Can you work these out from the model? Positions are in its coordinate system, mm. A direction names the side the tool comes from. Give positions to 0.01 mm unless a question says otherwise; leave off trailing zeros. Write each loop counter-clockwise with the first axis right and the second up, starting at its lowest first coordinate (ties: lowest second). Pieces come first, ordered by that corner, then holes. Notation, with made-up numbers: (62, 7.25) -> (119, 7.25) arc R33 ccw to (119, 45.25) -> close; hole circle Ø3 at (15.25, 20.25). An arc over 180 degrees is marked (long way). Answer as CSV lines item,"result". Start each with the question number.
1. If we mould it in two halves opening along X, with no side actions, what happens to faces 3 (the face through (66, 3, -50.8)), 4 (the face through (75.5, 3.1, 0.7)), 5 (the face through (3.175, 3, -13))? For each: pulls with the +X half, pulls with the -X half, needs draft (parallel to the pull), parting line crosses it, or undercut.
2. If we section it at A-A on z = 4.5: Write out the boundary of the cut face in (x, y) (3 decimals), plus the area to 3 significant figures.
3. I need wall thicknesses on line 1 (X direction, y = 5.75, z = 7.5) (3 decimals); line 2 (X direction, y = 5.5, z = -15) (3 decimals); line 3 (X direction, y = 3, z = 38). Which ranges of each line are inside material? Lowest first, please. Write a range as [from, to].
4. I'm going to push flat-ended pins straight in: P1, Ø3, axis at y = 4, z = -20, coming from the +X side; P2, Ø1.5, axis at y = 1, z = 34.5, coming from the +X side; P3, Ø1.9, axis at y = 3.5, z = -27, coming from the -X side. Where does each tip first touch, or does it pass through?
5. If we section it at D-D on x = -97: Write out the boundary of the cut face in (y, z), plus the area to 4 significant figures.
6. On a 3-axis mill with a long thin cutter (end or side, diameter ignored), from which of +Z, -Z, +X, -X, +Y, -Y can I reach the whole of each face in a straight line? I mean faces 1 (the face through (-3.175, 3, -12)), 2 (the face through (-26, 6.35, -12)). Say none if no direction works.
7. If we section it at B-B on y = 5: Write out the boundary of the cut face in (x, z) (3 decimals).
8. If we section it at C-C on z = -38.5: Write out the boundary of the cut face in (x, y) (3 decimals).
```python
from build123d import *

# Parameters (mm, degrees)
BOSS_EXTRUDE1_DEPTH = 6.35


with BuildPart() as part:
    # Sketch1 → Boss-Extrude1 (new body)
    with BuildSketch(Plane(origin=(0, 0, 0), x_dir=(1, 0, 0), z_dir=(0, 1, 0))):
        Polygon((-127, 50.8), (-25.4, 50.8), (-25.4, -50.8), align=None)
        with BuildLine():
            Line((-25.4, 50.8), (-25.4, -50.8))
            Line((-25.4, -50.8), (25.4, -50.8))
            Line((25.4, -50.8), (25.4, 50.8))
            Line((25.4, 50.8), (3.175, 50.8))
            Line((3.175, 50.8), (3.175, -25.4))
            ThreePointArc((3.175, -25.4), (0, -28.575), (-3.175, -25.4))
            Line((-3.175, -25.4), (-3.175, 50.8))
            Line((-3.175, 50.8), (-25.4, 50.8))
        make_face()
        Polygon((25.4, -50.8), (127, 50.8), (25.4, 50.8), align=None)
    extrude(amount=BOSS_EXTRUDE1_DEPTH)


solid = part.part
```
Computed values:
1,face 3,"needs draft"
1,face 4,"pulls with the +X half"
1,face 5,"undercut"
2,outline,"(-71.7, 0) -> (-3.175, 0) -> (-3.175, 6.35) -> (-71.7, 6.35) -> close; (3.175, 0) -> (71.7, 0) -> (71.7, 6.35) -> (3.175, 6.35) -> close"
2,area,"870 mm2"
3,line 1,"x = [-68.7, -3.175], [3.175, 68.7]"
3,line 2,"x = [-91.2, -3.175], [3.175, 91.2]"
3,line 3,"x = [-38.2, 38.2]"
4,P1,"stops at x = 97.7"
4,P2,"stops at x = 42.45"
4,P3,"stops at x = -104.15"
5,outline,"(0, -50.8) -> (6.35, -50.8) -> (6.35, -20.8) -> (0, -20.8) -> close"
5,area,"190.5 mm2"
6,face 1,"-Z, +Y, -Y"
6,face 2,"+Z, -Z, +X, -X, +Y"
7,outline,"(-127, -50.8) -> (-3.175, -50.8) -> (-3.175, 25.4) arc R3.175 cw to (3.175, 25.4) -> (3.175, -50.8) -> (127, -50.8) -> (25.4, 50.8) -> (-25.4, 50.8) -> close"
8,outline,"(-114.7, 0) -> (-3.175, 0) -> (-3.175, 6.35) -> (-114.7, 6.35) -> close; (3.175, 0) -> (114.7, 0) -> (114.7, 6.35) -> (3.175, 6.35) -> close"
